Check sheet for the modelled part. Datum: model origin and axes. Units: mm. A direction names the side the tool comes from. Give positions to 0.01 mm unless a question says otherwise; leave off trailing zeros. Write each loop counter-clockwise with the first axis right and the second up, starting at its lowest first coordinate (ties: lowest second). Pieces come first, ordered by that corner, then holes. Notation, with made-up numbers: (20.5, -24) -> (58.5, -24) arc R18 cw to (58.5, -12) -> close; hole circle Ø11 at (75.25, -36.5). An arc over 180 degrees is marked (long way). Write each question's results on one line, items separated by ' | '. Start each with the question number.
Autodesk Inventor part; units mm, degrees
ref_plane "Work Plane1" through (25, 0, -38.5) normal (0, 0, 1) x (1, 0, 0)
ref_plane "YZ Plane" through (0, 0, 0) normal (1, 0, 0) x (0, 1, 0)
ref_plane "XZ Plane" through (0, 0, 0) normal (0, 1, 0) x (-1, 0, 0)
sketch "Sketch1" plane through (0, 0, 0) normal (0, 1, 0) x (-1, 0, 0)
  line L0 (0, 0) -> (-50, 0)
  line L1 (-50, 0) -> (-50, -80)
  line L2 (-50, -80) -> (0, -80)
  line L3 (0, -80) -> (0, 0)
  circle A0 centre (-25, -80) radius 41.5
  point P0 (-50, -46.8752)
  point P1 (0, -46.8752)
  dimension "d0" = 50
  dimension "d1" = 83
  dimension "d14" = 80
extrude "Extrusion1" add sketch "Sketch1" along normal mid plane 60
sketch "Sketch2" plane through (0, 0, 0) normal (1, 0, 0) x (0, 1, 0)
  line L0 (30, 0) -> (-30, 0)
  circle A0 centre (0, 0) radius 30
extrude "Extrusion2" add sketch "Sketch2" along normal up to surface (50 mm away) contours L0 A0 picked at (-5.2341, 20.5501)
sketch "Sketch3" plane through (0, 30, 0) normal (0, 1, 0) x (1, 0, 0)
  arc A0 (50, 46.8752) -> (0, 46.8752) centre (25, 80) ccw
  circle A1 centre (25, 80) radius 41.5
  circle A2 centre (25, 80) radius 28
  line L0 (0, -30) -> (50, -30) construction
  line L1 (25, 80) -> (44.9219, 52.757) construction
  line L2 (8.1861, 50.8774) -> (25, 80) construction
  line L3 (50, 46.8752) -> (50, 47.5169)
  line L4 (0, 46.8752) -> (0, 0)
  line L5 (0, 46.8752) -> (0, 46.5678)
  circle A3 centre (25, 80) radius 33 construction
  line L6 (25, 80) -> (25, -30) construction
  line L7 (0, -30) -> (50, -30) construction
  arc A4 (11, 55.7513) -> (7.2217, 56.255) centre (8.5, 51.4212) ccw
  arc A5 (7.2217, 56.255) -> (0, 46.8752) centre (9.7022, 46.8752) ccw
  arc A6 (42.7783, 56.255) -> (39, 55.7513) centre (41.5, 51.4212) ccw
  arc A7 (50, 46.8752) -> (42.7783, 56.255) centre (40.2978, 46.8752) ccw
  point P0 (0, 46.8752)
  point P1 (66.5, 80)
  dimension "d15" = 56
  dimension "d22" = 66
  dimension "d23" = 30
extrude "Extrusion3" cut sketch "Sketch3" against normal blind 12.5 contours A7 A6 A2 A4 A5 A0 | A2
ref_plane "Work Plane1" through (25, 0, -38.5) normal (0, 0, 1) x (1, 0, 0)
sketch "Sketch4" plane through (25, 0, -38.5) normal (0, 0, 1) x (1, 0, 0)
  circle A0 centre (0, 0) radius 6
  line L0 (-14, 30) -> (14, 30) construction
  line L1 (0, 30) -> (0, -30) construction
  line L2 (-41.5, -30) -> (41.5, -30) construction
  line L3 (-25, 0) -> (25, 0) construction
  line L4 (25, -30) -> (25, 30) construction
  point P0 (-25, -30)
  point P1 (20.75, 17.5)
  point P2 (0, 0)
  dimension "d19" = 12
extrude "Extrusion4" cut sketch "Sketch4" along normal through all
properties part number "thigh_inventor"
Item 1: Section check A-A on y = 0. Record the boundary of the cut face in (x, z), then the cut area to 3 significant figures.
Item 2: Mould release check, pull along Y, two halves, no side actions. Record for faces 6 (the flat face through (24, 17.5, -85)), 7 (the flat face through (0, 0, -8)), 8 (the cylindrical face through (20.24, 3.65, -4.73)), 9 (the flat face through (26, -30, -60)): pulls with the +Y half, pulls with the -Y half, needs draft (parallel to the pull), parting line crosses it, or undercut.
Item 3: Thickness scan on probe 1 along X at (y, z) = (0, -19); probe 2 along Y at (x, z) = (25, -1); probe 3 along X at (y, z) = (17.5, -25). Record the ranges inside material, lowest first. Write a range as from..to.
Item 4: Depth check by flat-ended pin: pin 1 Ø2 at (y, z) = (19.5, 10.5) entering from -X; pin 2 Ø18 at (y, z) = (3, 8) entering from +X; pin 3 Ø2 at (x, z) = (-2.5, -14) entering from -Y; pin 4 Ø6 at (x, z) = (36.5, -61.5) entering from +Y. Enter the tip coordinate at first touch or a pass-through.
Item 5: Set-up check for faces 1 (the cylindrical face through (40.87, 23.84, -56.38)), 2 (the cylindrical face through (48.04, 23.84, -52.72)), 3 (the flat face through (50, 0, -8)), 4 (the cylindrical face through (2.069, 23.838, -52.864)), 5 (the flat face through (25, 0, -38.5)): record each of +Z, -Z, +X, -X, +Y, -Y from which the full face is reachable in a straight line by a thin tool's end or side.
Item 6: Section check D-D on z = -80. Record the boundary of the cut face in (x, y).
Item 7: Section check C-C on z = 11.5. Record the boundary of the cut face in (x, y), then the cut area to 3 significant figures.
Item 8: Section check B-B on x = 20.5. Record the boundary of the cut face in (y, z), then the cut area to 3 significant figures.
Check sheet entries:
1) outline: (0, -46.88) arc R41.5 ccw (long way) to (50, -46.88) -> (50, 30) -> (31, 30) -> (31, -38.5) -> (19, -38.5) -> (19, 30) -> (0, 30) -> close | area: 8,150 mm^2
2) face 6: pulls with the +Y half | face 7: needs draft | face 8: undercut | face 9: pulls with the -Y half
3) probe 1: x = 0..19, 31..50 | probe 2: y = -30..-6, 6..30 | probe 3: x = 0..50
4) pin 1: stops at x = 0 | pin 2: stops at x = 50 | pin 3: passes through | pin 4: stops at y = 17.5
5) face 1: -Z, +Y | face 2: -Z, +X, +Y | face 3: +Z, +X, +Y, -Y | face 4: -Z, -X, +Y | face 5: +Z
6) outline: (-16.5, -30) -> (66.5, -30) -> (66.5, 17.5) -> (-16.5, 17.5) -> close
7) outline: (0, -27.71) -> (50, -27.71) -> (50, 27.71) -> (0, 27.71) -> close; hole circle Ø12 at (25, 0) | area: 2,660 mm^2
8) outline: (-30, -121.26) -> (17.5, -121.26) -> (17.5, -52.36) -> (30, -52.36) -> (30, 0) arc R30 ccw to (3.97, 29.74) -> (3.97, -38.5) -> (-3.97, -38.5) -> (-3.97, 29.74) arc R30 ccw to (-30, 0) -> close | area: 7,280 mm^2
